Autodesk Inventor part; units mm, degrees
ref_plane "YZ Plane" through (0, 0, 0) normal (1, 0, 0) x (0, 1, 0)
ref_plane "XZ Plane" through (0, 0, 0) normal (0, 1, 0) x (-1, 0, 0)
ref_plane "XY Plane" through (0, 0, 0) normal (0, 0, 1) x (1, 0, 0)
sketch "Sketch1" plane through (0, 0, 0) normal (0, 0, 1) x (1, 0, 0)
  line L0 (-9, 10) -> (9, 10)
  line L1 (10, 9) -> (10, -9)
  line L2 (9, -10) -> (-9, -10)
  line L3 (-10, -9) -> (-10, 9)
  line L4 (-10, 10) -> (10, -10) construction
  line L5 (10, 10) -> (-10, -10) construction
  circle A0 centre (0, 0) radius 2
  line L6 (-4, 4) -> (4, 4)
  line L7 (4, 4) -> (4, -4)
  line L8 (4, -4) -> (-4, -4)
  line L9 (-4, -4) -> (-4, 4)
  line L10 (-4, 4) -> (4, -4) construction
  line L11 (4, 4) -> (-4, -4) construction
  arc A1 (-9, 10) -> (-10, 9) centre (-9, 9) ccw
  arc A2 (10, 9) -> (9, 10) centre (9, 9) ccw
  arc A3 (9, -10) -> (10, -9) centre (9, -9) ccw
  arc A4 (-10, -9) -> (-9, -10) centre (-9, -9) ccw
  line L12 (-3.1, 10) -> (3.1, 10)
  line L13 (3.1, 10) -> (3.1, -10)
  line L14 (3.1, -10) -> (-3.1, -10)
  line L15 (-3.1, -10) -> (-3.1, 10)
  line L16 (-10, 3.1) -> (10, 3.1)
  line L17 (10, 3.1) -> (10, -3.1)
  line L18 (10, -3.1) -> (-10, -3.1)
  line L19 (-10, -3.1) -> (-10, 3.1)
  line L20 (-5.5, 10) -> (5.5, 10)
  line L21 (5.5, 10) -> (5.5, -10)
  line L22 (5.5, -10) -> (-5.5, -10)
  line L23 (-5.5, -10) -> (-5.5, 10)
  line L24 (-10, 5.5) -> (10, 5.5)
  line L25 (10, 5.5) -> (10, -5.5)
  line L26 (10, -5.5) -> (-10, -5.5)
  line L27 (-10, -5.5) -> (-10, 5.5)
  line L28 (-8.3, 5.5) -> (-8.3, 3.1)
  line L29 (-8.3, -5.5) -> (-8.3, -3.1)
  line L30 (8.3, -5.5) -> (8.3, -3.1)
  line L31 (8.3, 5.5) -> (8.3, 3.1)
  line L32 (-5.5, 8.3) -> (-3.1, 8.3)
  line L33 (3.1, 8.3) -> (5.5, 8.3)
  line L34 (-5.5, -8.3) -> (-3.1, -8.3)
  line L35 (3.1, -8.3) -> (5.5, -8.3)
  line L36 (-4, 2.5) -> (-7, 5.5)
  line L37 (-4, 2.5) -> (0.2426, 2.5) construction
  line L38 (-4, -2.5) -> (-7, -5.5)
  line L39 (-4, -2.5) -> (0.2426, -2.5) construction
  line L40 (-2.5, 4) -> (-5.5, 7)
  line L41 (-2.5, 4) -> (1.7426, 4) construction
  line L42 (5.5, 7) -> (2.5, 4)
  line L43 (5.5, 7) -> (9.7426, 7) construction
  line L44 (7, 5.5) -> (4, 2.5)
  line L45 (7, 5.5) -> (11.2426, 5.5) construction
  line L46 (7, -5.5) -> (4, -2.5)
  line L47 (7, -5.5) -> (11.2426, -5.5) construction
  line L48 (2.5, -4) -> (5.5, -7)
  line L49 (2.5, -4) -> (6.7426, -4) construction
  line L50 (-2.5, -4) -> (-5.5, -7)
  line L51 (-2.5, -4) -> (1.7426, -4) construction
  point P0 (3.1, -3.1)
  point P1 (3.1, -5.5)
  point P2 (5.5, -5.5)
  point P3 (10, 3.1)
  point P4 (-5.5, -5.5)
  point P5 (-3.1, -5.5)
  point P6 (-3.1, -3.1)
  dimension "d0" = 20
  dimension "d1" = 20
  dimension "d2" = 4
  dimension "d3" = 8
  dimension "d4" = 8
  dimension "d5" = 1
  dimension "d6" = 6.2
  dimension "d7" = 3.1
  dimension "d8" = 6.2
  dimension "d9" = 3.1
  dimension "d10" = 11
  dimension "d11" = 5.5
  dimension "d12" = 11
  dimension "d13" = 5.5
  dimension "d14" = 4.3
  dimension "d15" = 4.3
  dimension "d16" = 4.3
  dimension "d17" = 4.3
  dimension "d18" = 135
  dimension "d19" = 135
  dimension "d20" = 135
  dimension "d21" = 135
  dimension "d22" = 135
  dimension "d23" = 135
  dimension "d24" = 1.3
  dimension "d25" = 1.3
  dimension "d26" = 1.3
  dimension "d27" = 1.3
  dimension "d28" = 1.3
  dimension "d29" = 1.3
  dimension "d32" = 45
  dimension "d33" = 135
  dimension "d34" = 1.3
  dimension "d35" = 1.3
extrude "Extrusion1" add sketch "Sketch1" along normal blind 90 contours L0 L23 L24 L3 A1 | L0 L15 L32 L23 | L24 L28 L16 L3 | L0 L21 L33 L13 | L40 L24 L23 | L0 A2 L1 L24 L21 | L24 L40 L15 L6 L9 L16 L36 L23 | L23 L36 L24 | L18 L29 L26 L3 | L40 L6 L15 | L26 L23 L2 A4 L3 | L21 L24 L42 | L42 L24 L21 L44 L16 L7 L6 L13 | L13 L6 L42 | L15 L16 L9 L6 | L6 L13 L16 L15 | L16 L9 L36 | L1 L16 L31 L24 | L24 L44 L21 | L6 L7 L16 L13 | L16 L13 L18 L15 | L15 L18 L9 L16 | L38 L23 L26 | L38 L9 L18 | L18 L9 L8 L15 L50 L26 L23 L38 | L16 L7 L18 L13 | L18 L13 L8 L15 | L15 L8 L9 L18 | L23 L34 L15 L2 | L26 L50 L23 | L1 L26 L30 L18 | L44 L7 L16 | L18 L7 L8 L13 | L8 L50 L15 | L1 A3 L2 L21 L26 | L13 L48 L8 | L8 L7 L18 L46 L21 L26 L48 L13 | L7 L46 L18 | L13 L35 L21 L2 | L46 L26 L21 | L21 L48 L26
equation "\"d7\" = 0.5 * d6"
equation "\"d8\" = d6"
equation "\"d11\" = 0.5 * d10"
equation "\"d12\" = d10"
properties part number "Aluminum_Profile_202090"
Work out the finished part from the listing and answer in its coordinate system (mm). A direction names the side the tool comes from. Coordinates: 2 decimals unless noted, no trailing zeros. Loops run counter-clockwise (first coordinate to the right, second up) from the corner with the lowest first, then second, coordinate; pieces in that order, holes last. Notation, with made-up numbers: M 74.5,-30 L 87.5,-30 A18 ccw 87.5,-8 Z; hole C -1.5,62 d1. An arc over 180 degrees is marked long. Answer in a Markdown table with one row per item. Add a question column.
1. A tool of negligible diameter and unlimited length cuts with its end or side. For faces 1 (the flat face through (-4, -5.5, 44.4)), 2 (the flat face through (-3.1, -9, 44)), 3 (the flat face through (-9, 3.1, 44)), from which of +Z, -Z, +X, -X, +Y, -Y can it reach the whole face along a straight path? Write none if from no direction.
2. The mould has two halves that part along Y. Classify faces 4 (the flat face through (-0.1, 2.4, 0)), 5 (the flat face through (4, -8.3, 44)), 6 (the flat face through (-6, -10, 44)): pulls with the +Y half, pulls with the -Y half, needs draft (parallel to the pull), parting line crosses it, or undercut.
3. Consider L1, parallel to X at y = 8, z = 46.5; L2, parallel to Y at x = 0, z = 52.5; L3, parallel to Y at x = 3.75, z = 65. Determine where each line is inside the solid, lowest interval first.
4. Flat-ended cylindrical pins translate along their axes: P1, Ø1.5, axis at y = 0, z = 33.5, coming from the +X side; P2, Ø2.5, axis at x = -1, z = 33.5, coming from the -Y side. Find the tip coordinate at first contact, or state that the pin passes through.
5. Find section A-A, the plane x = 0. Write down the section's boundary in (y, z), then the cut area to 3 significant figures.
Reported:
| question | item | result |
|---|---|---|
| 1 | face 1 | +Z, -Z |
| 1 | face 2 | +Z, -Z, -Y |
| 1 | face 3 | +Z, -Z, -X |
| 2 | face 4 | needs draft |
| 2 | face 5 | undercut |
| 2 | face 6 | pulls with the -Y half |
| 3 | L1 | x = -10 to -5.5, 5.5 to 10 |
| 3 | L2 | y = -4 to -2, 2 to 4 |
| 3 | L3 | y = -10 to -8.3, -5.25 to 5.25, 8.3 to 10 |
| 4 | P1 | stops at x = 4 |
| 4 | P2 | stops at y = -4 |
| 5 | outline | M -4,0 L -2,0 L -2,90 L -4,90 Z; M 2,0 L 4,0 L 4,90 L 2,90 Z |
| 5 | area | 360 mm^2 |
